The figure shows three views and two pictorial views of one solid part (mm, origin at its lowest corner). Answer the questions. Round coordinates to 2 decimals unless told otherwise and drop trailing zeros. Order: outer loops, then holes, each group sorted by start corner. A loop starts at its lowest first (then second) coordinate and runs counter-clockwise, first axis right, second up. Notation, with made-up numbers: (47.25, 69.25) - (62.25, 69.25) arc R19 cw to (62.25, 77.25) - close; hole circle Ø5 at (23, 27.5). An arc over 180 degrees is marked (long way). Use CSV: the item, a comma, the result in double quotes. Start each with the question number.
Item 1: Straight lines are drawn through the part: line 1 along Z through (x, y) = (710, 67); line 2 along X through (y, z) = (108, 609); line 3 along Z through (x, y) = (120, 115.5). For each, find the intervals that lie inside material, in ascending order. Write a range as [from, to].
Item 2: Find section B-B, the plane x = 710. Give the vertices of the cut face in (y, z), plus the area to 4 significant figures.
Item 3: Find section A-A, the plane z = 1350. Give the vertices of the cut face in (x, y).
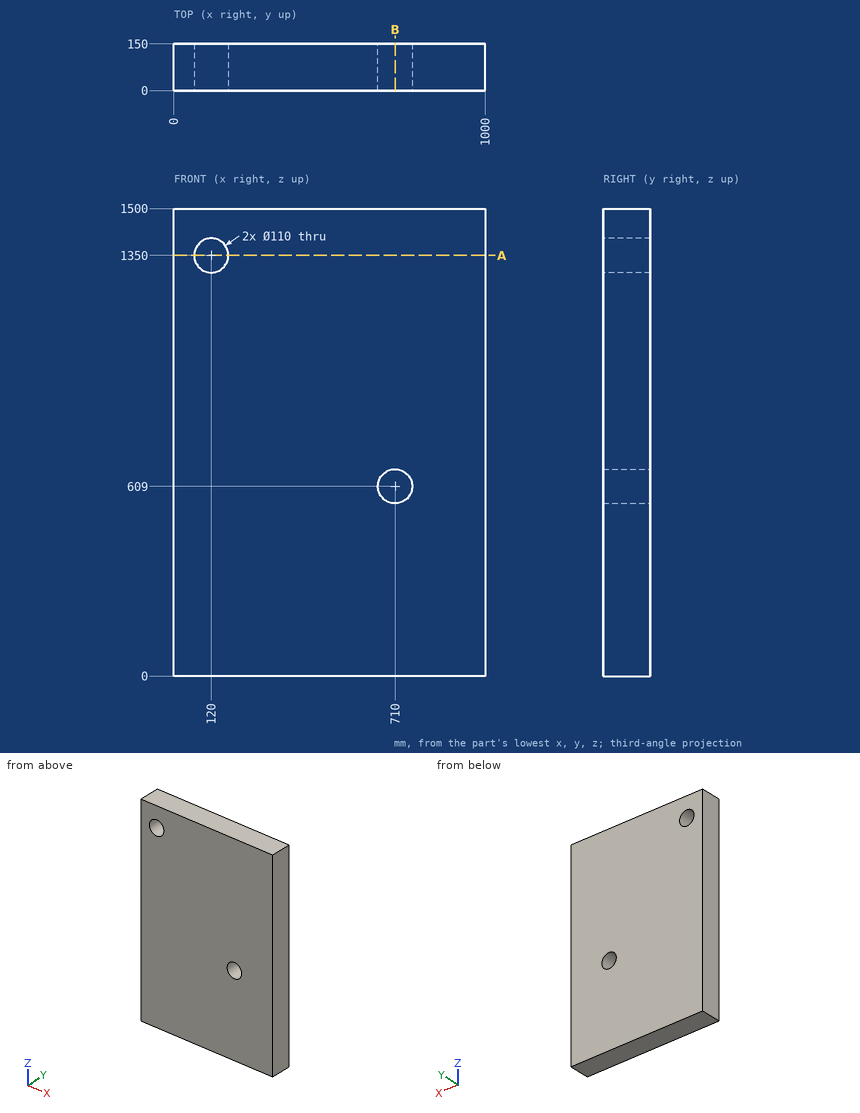
Worked out:
1,line 1,"z = [0, 554], [664, 1500]"
1,line 2,"x = [0, 655], [765, 1000]"
1,line 3,"z = [0, 1295], [1405, 1500]"
2,outline,"(0, 0) - (150, 0) - (150, 554) - (0, 554) - close; (0, 664) - (150, 664) - (150, 1500) - (0, 1500) - close"
2,area,"208,500 mm²"
3,outline,"(0, 0) - (65, 0) - (65, 150) - (0, 150) - close; (175, 0) - (1000, 0) - (1000, 150) - (175, 150) - close"
